from build123d import *

# Parameters (mm, degrees)
F2_DEPTH = 3
F1_W     = 10.2
F1_H     = 8.1991158426
F1_H_2   = 21.2707020342
F3_DEPTH = 3


with BuildPart() as f2:
    # F0 (on Top) → F2 (new body)
    with BuildSketch(Plane.XY):
        with BuildLine():
            ThreePointArc((11.3067825639, 29.4007936636), (11.4515937375, 30.4459601281), (11.4999999642, 31.5))
            ThreePointArc((11.4999999642, 31.5), (-1.0540399207, 42.9515937721), (-11.3067826307, 29.4007936379))
            ThreePointArc((-11.3067826307, 29.4007936379), (-3.58e-08, 31.5), (11.3067825639, 29.4007936636))
        make_face()
        with BuildLine():
            ThreePointArc((11.3067825639, 29.4007936636), (-3.58e-08, 31.5), (-11.3067826307, 29.4007936379))
            ThreePointArc((-11.3067826307, 29.4007936379), (-2.27e-08, 20), (11.3067825639, 29.4007936636))
        make_face()
        with BuildLine():
            ThreePointArc((11.3067825639, 29.4007936636), (-2.27e-08, 20), (-11.3067826307, 29.4007936379))
            ThreePointArc((-11.3067826307, 29.4007936379), (-27.2798002371, 15.749999969), (-31.1152254861, -4.9084358964))
            ThreePointArc((-31.1152254861, -4.9084358964), (-20.641178009, -6.3596488455), (-15.7798002013, -15.750000031))
            ThreePointArc((-15.7798002013, -15.750000031), (-16.8354091384, -20.5629716001), (-19.8084428665, -24.4923578123))
            ThreePointArc((-19.8084428665, -24.4923578123), (3.58e-08, -31.5), (19.8084429222, -24.4923577673))
            ThreePointArc((19.8084429222, -24.4923577673), (17.320508087, -9.9999999803), (31.1152254973, -4.9084358257))
            ThreePointArc((31.1152254973, -4.9084358257), (31.4036590477, -2.4617470256), (31.5, 0))
            ThreePointArc((31.5, 0), (25.965492974, 17.8337650152), (11.3067825639, 29.4007936636))
        make_face()
        with BuildLine():
            ThreePointArc((-19.8084428665, -24.4923578123), (-27.2798002013, -15.750000031), (-31.1152254861, -4.9084358964))
            ThreePointArc((-31.1152254861, -4.9084358964), (-37.2390923383, -21.5000000423), (-19.8084428665, -24.4923578123))
        make_face()
        with BuildLine():
            ThreePointArc((-15.7798002013, -15.750000031), (-20.641178009, -6.3596488455), (-31.1152254861, -4.9084358964))
            ThreePointArc((-31.1152254861, -4.9084358964), (-27.2798002013, -15.750000031), (-19.8084428665, -24.4923578123))
            ThreePointArc((-19.8084428665, -24.4923578123), (-16.8354091384, -20.5629716001), (-15.7798002013, -15.750000031))
        make_face()
        with BuildLine():
            ThreePointArc((19.8084429222, -24.4923577673), (27.2798002371, -15.749999969), (31.1152254973, -4.9084358257))
            ThreePointArc((31.1152254973, -4.9084358257), (17.320508087, -9.9999999803), (19.8084429222, -24.4923577673))
        make_face()
        with BuildLine():
            ThreePointArc((38.7798002371, -15.749999969), (36.6701514151, -9.111377766), (31.1152254973, -4.9084358257))
            ThreePointArc((31.1152254973, -4.9084358257), (27.2798002371, -15.749999969), (19.8084429222, -24.4923577673))
            ThreePointArc((19.8084429222, -24.4923577673), (32.0927718181, -26.1943910265), (38.7798002371, -15.749999969))
        make_face()
    extrude(amount=F2_DEPTH)

    # F1 (on Top) → F3 (cut)
    with BuildSketch(Plane.XY):
        with BuildLine():
            Line((5.1, 25), (5.1, 16.8008841574))
            Line((5.1, 16.8008841574), (-5.1, 16.8008841574))
            Line((-5.1, 16.8008841574), (-5.1, 25))
            Line((-5.1, 25), (-10, 25))
            ThreePointArc((-10, 25), (-20.6066017178, 20.6066017178), (-25, 10))
            Line((-25, 10), (-25, -10))
            ThreePointArc((-25, -10), (-20.6066017178, -20.6066017178), (-10, -25))
            Line((-10, -25), (10, -25))
            ThreePointArc((10, -25), (20.6066017178, -20.6066017178), (25, -10))
            Line((25, -10), (25, 10))
            ThreePointArc((25, 10), (20.6066017178, 20.6066017178), (10, 25))
            Line((10, 25), (5.1, 25))
        make_face()
        with Locations((0, 20.9004420787)):
            Rectangle(F1_W, F1_H)
        with Locations((0, 35.6353510171)):
            Rectangle(F1_W, F1_H_2)
    extrude(amount=F3_DEPTH, mode=Mode.SUBTRACT)


solid = f2.part
Verification items for the finished model (mm, model axes). A direction names the side the tool comes from. Coordinates: 2 decimals unless noted, no trailing zeros. Order: outer loops, then holes, each group sorted by start corner. A loop starts at its lowest first (then second) coordinate and runs counter-clockwise, first axis right, second up.
1. Set-up check for faces 5 (the face through (-5.1, 33, 1)), 6 (the face through (0, -27, 3)), 7 (the face through (8, 25, 1)): record each of +Z, -Z, +X, -X, +Y, -Y from which the full face is reachable in a straight line by a thin tool's end or side.
Results found:
face 5: +Z, -Z, +Y
face 6: +Z, +X, -X, +Y, -Y
face 7: +Z, -Z
2. Sectioned sample at A-A, the plane y = 6. Record the cut outline in (x, z).
Results found:
outline: (-30.92, 0) - (-25, 0) - (-25, 3) - (-30.92, 3) - close; (25, 0) - (30.92, 0) - (30.92, 3) - (25, 3) - close
3. Go/stop test with flat-tipped pins: pin 1 Ø1.5 at (y, z) = (2, 2) entering from +X; pin 2 Ø1.5 at (x, z) = (6.5, 1.5) entering from -Y; pin 3 Ø0.9 at (y, z) = (1.5, 1.5) entering from -X. Record where each tip stops, or that it passes through.
Results found:
pin 1: stops at x = 31.48
pin 2: stops at y = -30.97
pin 3: stops at x = -31.48
4. Sectioned sample at D-D, the plane x = -28. Record the cut outline in (y, z).
Results found:
outline: (-27.23, 0) - (14.43, 0) - (14.43, 3) - (-27.23, 3) - close
5. Sectioned sample at B-B, the plane x = 6. Record the cut outline in (y, z), and give its area (3 significant figures).
Results found:
outline: (-30.92, 0) - (-25, 0) - (-25, 3) - (-30.92, 3) - close; (25, 0) - (41.31, 0) - (41.31, 3) - (25, 3) - close
area: 66.7 mm2
6. Scan lines: line 1 (X direction, y = 32, z = 0.2); line 2 (X direction, y = 33, z = 1.15); line 3 (Y direction, x = 20.5, z = 1.2). Record each from-to range of solid material in increasing order.
Results found:
line 1: x = -11.49 to -5.1, 5.1 to 11.49
line 2: x = -11.4 to -5.1, 5.1 to 11.4
line 3: y = -25.04 to -20.71, 20.71 to 23.92
7. Sectioned sample at C-C, the plane z = 2.5. Record the cut outline in (x, y).
Results found:
outline: (-31.12, -4.91) arc R11.5 ccw (long way) to (-19.81, -24.49) arc R31.5 ccw to (19.81, -24.49) arc R11.5 ccw (long way) to (31.12, -4.91) arc R31.5 ccw to (11.31, 29.4) arc R11.5 ccw to (5.1, 41.81) - (5.1, 25) - (10, 25) arc R15 cw to (25, 10) - (25, -10) arc R15 cw to (10, -25) - (-10, -25) arc R15 cw to (-25, -10) - (-25, 10) arc R15 cw to (-10, 25) - (-5.1, 25) - (-5.1, 41.81) arc R11.5 ccw to (-11.31, 29.4) arc R31.5 ccw to start
8. Release check for a two-part mould opening along Y. For faces 1 (the face through (-20.49, 20.72, 1.48)), 2 (the face through (5.1, 33, 1)), 3 (the face through (20.72, 20.49, 1.48)), 4 (the face through (-0.3, -31.5, 1.5)) record: +Y half, -Y half, draft (parallel to the pull), parting line (faces both ways), or undercut.
Results found:
face 1: undercut
face 2: draft
face 3: undercut
face 4: -Y half
